Design review of the part built by this model. Coordinates are the model's own, in mm. Round coordinates to 2 decimals unless told otherwise and drop trailing zeros. Loops run counter-clockwise (first coordinate to the right, second up) from the corner with the lowest first, then second, coordinate; pieces in that order, holes last. Notation, with made-up numbers: (-17.5, 59.25) - (11.5, 59.25) arc R20 ccw to (11.5, 82.25) - close; hole circle Ø3 at (7.5, 5). An arc over 180 degrees is marked (long way). Use one line per item in the form item = value. Start each with the question number.
(1) We need section B-B, the plane z = 75. Write out the cut boundary in (x, y), then the cut area to 3 significant figures.
(2) For pin 1 (4 mm diameter, centred on x = 27.5, z = 34, fed in from -Y), flat-tipped, find the tip position at first contact; note if it passes through.
(3) We need section A-A, the plane x = 75. Write out the cut boundary in (y, z), then the cut area to 3 significant figures.
(4) We need section C-C, the plane y = 2.3. Give the number of separate pieces and of enclosed holes in the cut face, then the cut area to 3 significant figures.
(5) Wall thickness on probe 1 along X at (y, z) = (0.25, -0.5); probe 2 along Z at (x, y) = (79.5, 1.9); probe 3 along Z at (x, y) = (26.5, 1.75): over which ranges is each line inside the solid? List them lowest first. Write a range as [from, to].
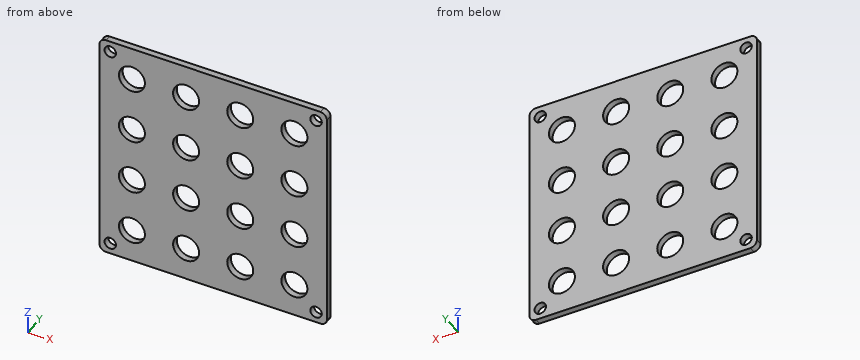
from build123d import *

# Parameters (mm, degrees)
SKETCH1_W            = 105
SKETCH1_H            = 105
SKETCH1_R            = 6
BOSS_EXTRUDE1_DEPTH  = 3
M5_CLEARANCE_HOLE1_D = 5.3
FILLET2_R            = 3


with BuildPart() as part:
    # Sketch1 → Boss-Extrude1 (new body)
    with BuildSketch(Plane(origin=(0, 0, 0), x_dir=(1, 0, 0), z_dir=(0, 1, 0))):
        with Locations((37.5, -37.5)):
            Rectangle(SKETCH1_W, SKETCH1_H)
        with Locations(Location((0, 0, 0), (0, 0, 270))):
            Circle(SKETCH1_R, mode=Mode.SUBTRACT)
        with Locations(Location((25, 0, 0), (0, 0, 270))):
            Circle(SKETCH1_R, mode=Mode.SUBTRACT)
        with Locations(Location((50, 0, 0), (0, 0, 270))):
            Circle(SKETCH1_R, mode=Mode.SUBTRACT)
        with Locations(Location((75, 0, 0), (0, 0, 270))):
            Circle(SKETCH1_R, mode=Mode.SUBTRACT)
        with Locations(Location((25, -25, 0), (0, 0, 270))):
            Circle(SKETCH1_R, mode=Mode.SUBTRACT)
        with Locations(Location((50, -25, 0), (0, 0, 270))):
            Circle(SKETCH1_R, mode=Mode.SUBTRACT)
        with Locations(Location((75, -25, 0), (0, 0, 270))):
            Circle(SKETCH1_R, mode=Mode.SUBTRACT)
        with Locations(Location((25, -50, 0), (0, 0, 270))):
            Circle(SKETCH1_R, mode=Mode.SUBTRACT)
        with Locations(Location((50, -50, 0), (0, 0, 270))):
            Circle(SKETCH1_R, mode=Mode.SUBTRACT)
        with Locations(Location((75, -50, 0), (0, 0, 270))):
            Circle(SKETCH1_R, mode=Mode.SUBTRACT)
        with Locations(Location((0, -25, 0), (0, 0, 270))):
            Circle(SKETCH1_R, mode=Mode.SUBTRACT)
        with Locations(Location((0, -50, 0), (0, 0, 270))):
            Circle(SKETCH1_R, mode=Mode.SUBTRACT)
        with Locations(Location((0, -75, 0), (0, 0, 270))):
            Circle(SKETCH1_R, mode=Mode.SUBTRACT)
        with Locations(Location((75, -75, 0), (0, 0, 270))):
            Circle(SKETCH1_R, mode=Mode.SUBTRACT)
        with Locations(Location((25, -75, 0), (0, 0, 270))):
            Circle(SKETCH1_R, mode=Mode.SUBTRACT)
        with Locations(Location((50, -75, 0), (0, 0, 270))):
            Circle(SKETCH1_R, mode=Mode.SUBTRACT)
    extrude(amount=BOSS_EXTRUDE1_DEPTH)

    # M5 Clearance Hole1 (through all)
    with Locations(Plane(origin=(0, 3, 0), x_dir=(1, 0, 0), z_dir=(0, 1, 0))):
        with Locations((-10, 10), (-10, -85), (85, -85), (85, 10)):
            Hole(M5_CLEARANCE_HOLE1_D / 2)

    # Fillet2
    fillet2_edges = [part.edges().sort_by_distance(p)[0] for p in [
        (-15, 1.5, -15),
        (90, 1.5, -15),
        (90, 1.5, 90),
        (-15, 1.5, 90),
    ]]
    fillet(fillet2_edges, radius=FILLET2_R)


solid = part.part
Data:
q1.outline = (-15, 0) - (-6, 0) - (-6, 3) - (-15, 3) - close; (6, 0) - (19, 0) - (19, 3) - (6, 3) - close; (31, 0) - (44, 0) - (44, 3) - (31, 3) - close; (56, 0) - (69, 0) - (69, 3) - (56, 3) - close; (81, 0) - (90, 0) - (90, 3) - (81, 3) - close
q1.area = 171 mm^2
q2.pin_1 = 0
q3.outline = (0, -15) - (3, -15) - (3, -6) - (0, -6) - close; (0, 6) - (3, 6) - (3, 19) - (0, 19) - close; (0, 31) - (3, 31) - (3, 44) - (0, 44) - close; (0, 56) - (3, 56) - (3, 69) - (0, 69) - close; (0, 81) - (3, 81) - (3, 90) - (0, 90) - close
q3.area = 171 mm^2
q4.separate_pieces = 1
q4.enclosed_holes = 20
q4.area = 9,120 mm^2
q5.probe_1 = [-15, -5.98], [5.98, 19.02], [30.98, 44.02], [55.98, 69.02], [80.98, 90]
q5.probe_2 = [-15, -3.97], [3.97, 21.03], [28.97, 46.03], [53.97, 71.03], [78.97, 90]
q5.probe_3 = [-15, -5.81], [5.81, 19.19], [30.81, 44.19], [55.81, 69.19], [80.81, 90]
